from build123d import *

# Parameters (mm, degrees)
F1_DEPTH = 20
F2_R     = 2.15
F3_DEPTH = 5


with BuildPart() as f1:
    # F0 (on Top) → F1 (new body)
    with BuildSketch(Plane.XY):
        Polygon((42.720473, 33.887387), (-27.279527, 33.887387), (-27.279527, 23.887387), (37.720473, 23.887387), align=None)
    extrude(amount=F1_DEPTH)

    # F2 (on face) → F3 (join)
    with BuildSketch(Plane.XY.offset(20)):
        with Locations((-22.207731, 28.838353)):
            Circle(F2_R)
        with Locations((29.88103, 28.887387)):
            Circle(F2_R)
    extrude(amount=F3_DEPTH)


solid = f1.part
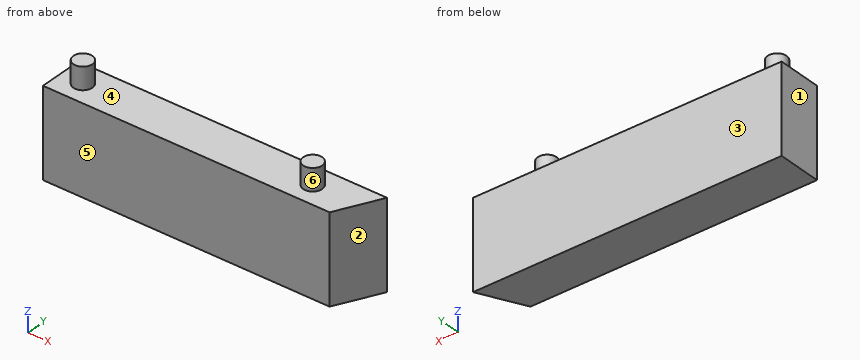
Source: CAD feature listing. Evaluate the final solid. Frame: model axes, mm. Face numbers are marked on the shaded views. A direction names the side the tool comes from. Coordinates: 2 decimals unless noted, no trailing zeros. Loops run counter-clockwise (first coordinate to the right, second up) from the corner with the lowest first, then second, coordinate; pieces in that order, holes last. Notation, with made-up numbers: (38, -29.75) - (48, -29.75) arc R23 cw to (48, -1.75) - close; hole circle Ø10 at (1.25, 5.25). An arc over 180 degrees is marked (long way). One line per question, with ' | ' between items.
1) Pull-direction query (X, two-part tool) for the marked faces 1, 2, 3 and 4; classes: released by +X, released by -X, zero draft, split by the parting line, or undercut.
Report:
face 1: released by -X | face 2: released by +X | face 3: zero draft | face 4: undercut
2) Section B-B, the plane z = 8.5. Return loops of the section in (x, y), then the cut area to 3 significant figures.
Report:
outline: (-27.28, 23.89) - (37.72, 23.89) - (42.72, 33.89) - (-27.28, 33.89) - close | area: 675 mm²
3) Set-up query: the marked faces 5 and 6. Return all of +Z, -Z, +X, -X, +Y, -Y with unobstructed straight access to the full face (end or side cutting, diameter ignored); none if empty.
Report:
face 5: +Z, -Z, +X, -X, -Y | face 6: +Z
4) Section A-A, the plane y = 29.5. Return loops of the section in (x, z).
Report:
outline: (-27.28, 0) - (40.53, 0) - (40.53, 20) - (31.94, 20) - (31.94, 25) - (27.82, 25) - (27.82, 20) - (-20.16, 20) - (-20.16, 25) - (-24.25, 25) - (-24.25, 20) - (-27.28, 20) - close
5) Section C-C, the plane x = -19. Return loops of the section in (y, z), then the cut area to 3 significant figures.
Report:
outline: (23.89, 0) - (33.89, 0) - (33.89, 20) - (23.89, 20) - close | area: 200 mm²
6) Line query: line 1 along Z through (x, y) = (-1, 30.75); line 2 along X through (y, z) = (30, 12.25); line 3 along X through (y, z) = (30.5, 18.75). Output: solid intervals per line, ascending.
Report:
line 1: z = 0 to 20 | line 2: x = -27.28 to 40.78 | line 3: x = -27.28 to 41.03
7) First-contact query: P1, Ø3, axis at x = 33.5, y = 30.5, coming from the +Z side; P2, Ø2, axis at y = 30.5, z = 18, coming from the +X side. Flat tips, straight axial feed; report the tip coordinate or a pass-through.
Report:
P1: stops at z = 20 | P2: stops at x = 41.53
